Model file for the job. Use its own axes, mm. A direction names the side the tool comes from. Round coordinates to 2 decimals unless told otherwise and drop trailing zeros. Order: outer loops, then holes, each group sorted by start corner. A loop starts at its lowest first (then second) coordinate and runs counter-clockwise, first axis right, second up. Notation, with made-up numbers: (84, 77) - (115, 77) arc R20 ccw to (115, 99) - close; hole circle Ø11 at (-23.5, -34.75). An arc over 180 degrees is marked (long way). Write item = value, one per line.
```python
from build123d import *

# Parameters (mm, degrees)
BOSS_EXTRUDE1_DEPTH = 31.75
FILLET3_R           = 12.7
FILLET1_SIZE        = 9.525
FILLET1_SIZE_2      = 6.35
FILLET2_R           = 2.54
SKETCH3_R           = 2.54
CUT_EXTRUDE1_DEPTH  = 48.161309524
SKETCH4_R           = 2.54
CUT_EXTRUDE2_DEPTH  = 45.901280775
CHAMFER1_SIZE       = 1.905


with BuildPart() as part:
    # Sketch1 → Boss-Extrude1 (new body)
    with BuildSketch(Plane(origin=(0, 0, 0), x_dir=(0, 0, -1), z_dir=(1, 0, 0))):
        Polygon((0, 0), (0, 25.4), (-19.05, 25.4), (-19.05, 29.21), (3.81, 29.21), (3.81, 0), align=None)
    extrude(amount=BOSS_EXTRUDE1_DEPTH)

    # Fillet3
    fillet3_edges = [part.edges().sort_by_distance(p)[0] for p in [
        (31.75, 27.305, 19.05),
        (31.75, 0, -1.905),
        (0, 27.305, 19.05),
        (0, 0, -1.905),
    ]]
    fillet(fillet3_edges, radius=FILLET3_R)

    # Fillet1
    # an asymmetric fillet: 9.525, 6.35 mm, written as the material it adds along each edge
    with BuildSketch(Plane(origin=(0, 25.4, 0), x_dir=(0, -1, 0), z_dir=(1, 0, 0))) as fillet1_piece_1:
        with BuildLine():
            Bezier((FILLET1_SIZE, 0), (0, 0), (0, -FILLET1_SIZE_2), weights=[1, 0.707106781, 1])
            Line((0, -FILLET1_SIZE_2), (0, 0))
            Line((0, 0), (FILLET1_SIZE, 0))
        make_face()
    extrude(amount=31.75)

    # Fillet2
    fillet2_edges = [part.edges().sort_by_distance(p)[0] for p in [
        (15.875, 0, 0),
        (15.875, 25.4, 19.05),
        (28.030256121, 25.4, 15.330256121),
        (31.75, 21.935812925, 1.451375627),
        (31.75, 14.2875, 0),
        (28.030256121, 3.719743879, 0),
        (3.719743879, 3.719743879, 0),
        (0, 14.2875, 0),
        (0, 21.935812925, 1.451375627),
        (3.719743879, 25.4, 15.330256121),
    ]]
    fillet(fillet2_edges, radius=FILLET2_R)

    # Sketch3 → Cut-Extrude1 (cut, through all)
    with BuildSketch(Plane.XY):
        with Locations((15.875, 9.2075)):
            Circle(SKETCH3_R)
    extrude(amount=-CUT_EXTRUDE1_DEPTH, mode=Mode.SUBTRACT)

    # Sketch4 → Cut-Extrude2 (cut, through all)
    with BuildSketch(Plane.XZ.offset(-25.4)):
        with Locations(Location((15.875, 11.43, 0), (0, 0, 270))):
            Circle(SKETCH4_R)
    extrude(amount=-CUT_EXTRUDE2_DEPTH, mode=Mode.SUBTRACT)

    # Chamfer1
    chamfer1_edges = [part.edges().sort_by_distance(p)[0] for p in [
        (15.875, 29.21, -3.81),
        (13.335, 9.2075, 0),
        (15.875, 25.4, 13.97),
    ]]
    chamfer(chamfer1_edges, length=CHAMFER1_SIZE)


solid = part.part
```
1) 3-axis set-ups, long thin cutter, end or side, ignore diameter. For faces 4 (the face through (0.764, 14.265, -0.724)), 5 (the face through (31.75, 24, -1)), 6 (the face through (30.986, 14.31, -0.724)), 7 (the face through (27.93, 28.58, 15.43)), 8 (the face through (19, 14, 0)): which of +Z, -Z, +X, -X, +Y, -Y reach the whole face in a straight line?
Conclusion:
face_4 = +Z, -X, -Y
face_5 = +Z, -Z, +X, +Y, -Y
face_6 = +Z, +X, -Y
face_7 = +Z, +X, +Y, -Y
face_8 = +Z, +X, -X, -Y
2) Wall check: line 1 along Z through (x, y) = (24, 11.5); line 2 along X through (y, z) = (28, 11.43) (3 decimals); line 3 along Y through (x, z) = (17.5, 7). Give the ranges that are in metal, low to high.
Conclusion:
line_1 = -3.81 to 0
line_2 = 1.06 to 13.335, 18.415 to 30.69
line_3 = 25.4 to 29.21
3) Cut at A-A (y = 14.75). Write the cut outline in (x, z).
Conclusion:
outline = (0, -3.81) - (31.75, -3.81) - (31.75, -2.54) arc R2.54 ccw to (29.21, 0) - (2.54, 0) arc R2.54 ccw to (0, -2.54) - close
4) Flat gauge pins, fed straight in: pin 1 Ø4 at (y, z) = (6.5, 0) entering from -X; pin 2 Ø1.5 at (x, z) = (12.5, 0.5) entering from -Y; pin 3 Ø5 at (x, z) = (11, 11.5) entering from -Y. Where does each tip first touch, or does it go through?
Conclusion:
pin_1 = 1.22
pin_2 = 1.44
pin_3 = 25.4
5) Mould opens along X. For faces 1 (the face through (15.7, 29.21, 8.7)), 2 (the face through (13.4, 28.2, 12)), 3 (the face through (0, 24, -1)) say: +X half, -X half, draft (parallel to the pull), parting line (faces both ways), or undercut.
Conclusion:
face_1 = draft
face_2 = undercut
face_3 = -X half
6) Cut at B-B (x = 14). Give the number of separate pieces and of enclosed holes in the cut face, and give its area (3 significant figures).
Conclusion:
separate_pieces = 3
enclosed_holes = 0
area = 157 mm^2
